```python
from build123d import *

# Parameters (mm, degrees)
SKETCH2_R           = 4.7625
BOSS_EXTRUDE1_DEPTH = 19.05
SKETCH3_R           = 4.7625
CUT_EXTRUDE1_DEPTH  = 139.7


with BuildPart() as part:
    # Sketch2 → Boss-Extrude1 (new body)
    with BuildSketch(Plane.XY):
        with BuildLine():
            Line((-63.5, 38.1), (63.5, 38.1))
            Line((63.5, 38.1), (63.5, -28.575))
            ThreePointArc((63.5, -28.575), (60.710192091, -35.310192091), (53.975, -38.1))
            Line((53.975, -38.1), (-53.975, -38.1))
            ThreePointArc((-53.975, -38.1), (-60.710192091, -35.310192091), (-63.5, -28.575))
            Line((-63.5, -28.575), (-63.5, 38.1))
        make_face()
        with Locations(Location((-44.45, -19.05, 0), (0, 0, 180))):
            Circle(SKETCH2_R, mode=Mode.SUBTRACT)
        with Locations(Location((44.45, -19.05, 0), (0, 0, 180))):
            Circle(SKETCH2_R, mode=Mode.SUBTRACT)
    extrude(amount=BOSS_EXTRUDE1_DEPTH)

    # Sketch3 → Cut-Extrude1 (cut)
    with BuildSketch(Plane(origin=(63.5, 0, 0), x_dir=(0, 0, -1), z_dir=(1, 0, 0))):
        with Locations((-9.525, 25.4)):
            Circle(SKETCH3_R)
    extrude(amount=-CUT_EXTRUDE1_DEPTH, mode=Mode.SUBTRACT)


solid = part.part
```
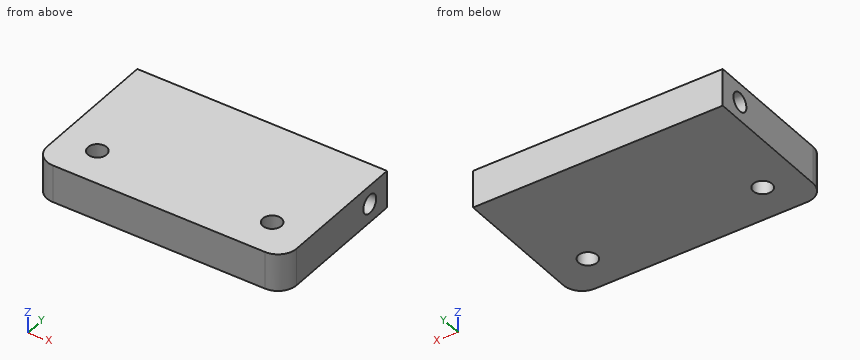
Here's how the part is built. I have some questions about the finished solid (model axes, mm). Coordinates: 2 decimals unless noted, no trailing zeros. Order: outer loops, then holes, each group sorted by start corner. A loop starts at its lowest first (then second) coordinate and runs counter-clockwise, first axis right, second up. Notation, with made-up numbers: (-35.5, -35.5) - (23.5, -35.5) arc R10 ccw to (23.5, -29.5) - close; hole circle Ø5 at (-31, 61.5). An arc over 180 degrees is marked (long way). One line per question, with ' | ' between items. Start each with the question number.
1. I'm going to push a flat-ended pin straight in: pin 1 Ø7.5 at (x, y) = (44.45, -19.05) entering from -Z. Where does the tip first touch, or does it pass through?
2. If we section it at B-B (y = -19.05): Write out the boundary of the cut face in (x, z).
3. If we section it at A-A (x = 44.45): Give the number of separate pieces and of enclosed holes in the cut face, and give its area (3 significant figures).
4. Please list where these lines run through material, in increasing order: line 1 along X through (y, z) = (-19.05, 5.5); line 2 along Z through (x, y) = (37, 25); line 3 along X through (y, z) = (-16, 2). Write a range as [from, to].
Model answer:
1) pin 1: passes through
2) outline: (-63.5, 0) - (-49.21, 0) - (-49.21, 19.05) - (-63.5, 19.05) - close; (-39.69, 0) - (39.69, 0) - (39.69, 19.05) - (-39.69, 19.05) - close; (49.21, 0) - (63.5, 0) - (63.5, 19.05) - (49.21, 19.05) - close
3) separate pieces: 2 | enclosed holes: 1 | area: 1,200 mm²
4) line 1: x = [-63.5, -49.21], [-39.69, 39.69], [49.21, 63.5] | line 2: z = [0, 4.78], [14.27, 19.05] | line 3: x = [-63.5, -48.11], [-40.79, 40.79], [48.11, 63.5]
